```python
from build123d import *

# Parameters (mm, degrees)
SKETCH_1_R          = 12
EXTRUDE_1_DEPTH     = 4
SKETCH_2_R          = 4
CUT_EXTRUDE_1_DEPTH = 9
SKETCH_3_R          = 10.3
SKETCH_3_R_2        = 7.05
CUT_EXTRUDE_2_DEPTH = 0.5


with BuildPart() as part:
    # 草圖1 → 填料-伸長1 (new body, symmetric)
    with BuildSketch(Plane.XY):
        Circle(SKETCH_1_R)
    extrude(amount=EXTRUDE_1_DEPTH, both=True)

    # 草圖2 → 除料-伸長1 (cut, through all)
    with BuildSketch(Plane.XY.offset(4)):
        Circle(SKETCH_2_R)
    extrude(amount=-CUT_EXTRUDE_1_DEPTH, mode=Mode.SUBTRACT)

    # 草圖3 → 除料-伸長2 (cut)
    with BuildSketch(Plane.XY.offset(4)):
        Circle(SKETCH_3_R)
        Circle(SKETCH_3_R_2, mode=Mode.SUBTRACT)
    cut_extrude_2 = extrude(amount=-CUT_EXTRUDE_2_DEPTH, mode=Mode.SUBTRACT)

    # 鏡射1: 除料-伸長2 across plane
    add(cut_extrude_2.mirror(Plane.XY), mode=Mode.SUBTRACT)


solid = part.part
```
Design review of the part built by this model. Coordinates are the model's own, in mm. A direction names the side the tool comes from. Coordinates: 2 decimals unless noted, no trailing zeros. Loops run counter-clockwise (first coordinate to the right, second up) from the corner with the lowest first, then second, coordinate; pieces in that order, holes last. Notation, with made-up numbers: (35.5, 32) -> (83.5, 32) arc R29 cw to (83.5, 64) -> close; hole circle Ø3 at (61.5, -37). An arc over 180 degrees is marked (long way). Answer as a JSON object with one key per item and string values.
Q1. Take a section at D-D on x = 9. Give the boundary of the cut face in (y, z), plus the area to 3 significant figures.
Answer block:
{"outline": "(-7.94, -4) -> (-5.01, -4) -> (-5.01, -3.5) -> (5.01, -3.5) -> (5.01, -4) -> (7.94, -4) -> (7.94, 4) -> (5.01, 4) -> (5.01, 3.5) -> (-5.01, 3.5) -> (-5.01, 4) -> (-7.94, 4) -> close", "area": "117 mm^2"}
Q2. Clearance check with flat-ended pins moving along their axes: pin 1 Ø4 at (x, y) = (5, -7.5) entering from -Z; pin 2 Ø2 at (y, z) = (-2.5, 2) entering from +X; pin 3 Ø2 at (y, z) = (-9, 0.5) entering from +X; pin 4 Ø3 at (x, z) = (-2.5, 0) entering from +Y. State where each tip first meets the part, or that it passes through.
Answer block:
{"pin 1": "stops at z = -4", "pin 2": "stops at x = 11.91", "pin 3": "stops at x = 8.94", "pin 4": "stops at y = 11.96"}
Q3. Take a section at C-C on z = -1.5. Give the boundary of the cut face in (x, y), plus the area to 3 significant figures.
Answer block:
{"outline": "circle Ø24 at (0, 0); hole circle Ø8 at (0, 0)", "area": "402 mm^2"}
Q4. Tool access review of faces 4 (the flat face through (-4, 10, 4)), 5 (the cylindrical face through (9.824, 3.094, 3.754)), 6 (the cylindrical face through (3.253, -6.255, -3.754)): name each direction out of +Z, -Z, +X, -X, +Y, -Y from which nothing blocks a thin tool from reaching the whole face with its end or side.
Answer block:
{"face 4": "+Z, +X, -X, +Y, -Y", "face 5": "+Z", "face 6": "-Z"}
Q5. Take a section at A-A on x = 0. Give the boundary of the cut face in (y, z).
Answer block:
{"outline": "(-12, -4) -> (-10.3, -4) -> (-10.3, -3.5) -> (-7.05, -3.5) -> (-7.05, -4) -> (-4, -4) -> (-4, 4) -> (-7.05, 4) -> (-7.05, 3.5) -> (-10.3, 3.5) -> (-10.3, 4) -> (-12, 4) -> close; (4, -4) -> (7.05, -4) -> (7.05, -3.5) -> (10.3, -3.5) -> (10.3, -4) -> (12, -4) -> (12, 4) -> (10.3, 4) -> (10.3, 3.5) -> (7.05, 3.5) -> (7.05, 4) -> (4, 4) -> close"}
Q6. To check wall thickness, follow L1, parallel to Y at x = 0, z = 3.75; L2, parallel to X at y = -0.25, z = -1.75; L3, parallel to Z at x = -9.75, y = -1.75. State the ranges of each line that lie inside material, in increasing order.
Answer block:
{"L1": "y = -12 to -10.3, -7.05 to -4, 4 to 7.05, 10.3 to 12", "L2": "x = -12 to -3.99, 3.99 to 12", "L3": "z = -3.5 to 3.5"}
Q7. The part is to be moulded in two halves that separate along X. For faces 1 (the flat face through (3, -3, 4)), 2 (the cylindrical face through (-11.99, 0.53, 0.06)), 3 (the cylindrical face through (9.824, 3.094, -3.754)), say which applies: +X half, -X half, draft (parallel to the pull), parting line (faces both ways), or undercut.
Answer block:
{"face 1": "draft", "face 2": "parting line", "face 3": "undercut"}
